from build123d import *

# Parameters (mm, degrees)
F0_W           = 31.095594
F0_H           = 13.626158
F3_D           = 6.35
F3_CSINK_D     = 12.7
F3_CSINK_ANGLE = 90


with BuildPart() as f1:
    # F0 (on Front) → F1 (revolve)
    with BuildSketch(Plane.XZ):
        with Locations((-50.311968, 6.813079)):
            Rectangle(F0_W, F0_H)
    revolve(axis=Axis((0, 0, -5.066134), (0, 0, -1)))

    # F3 (through all)
    with Locations(Plane(origin=(0, 0, 0), x_dir=(1, 0, 0), z_dir=(0, 0, -1))):
        with Locations((55.552796, 0), (0, 55.552796), (-55.552796, 0), (0, -55.552796)):
            CounterSinkHole(F3_D / 2, F3_CSINK_D / 2, counter_sink_angle=F3_CSINK_ANGLE)


solid = f1.part
Input: part model. Units: mm. Frame: model coordinates. Round coordinates to 2 decimals unless told otherwise and drop trailing zeros. Order: outer loops, then holes, each group sorted by start corner. A loop starts at its lowest first (then second) coordinate and runs counter-clockwise, first axis right, second up.
1. Mould query, pull axis Y, two halves, no side actions, for faces 1 (the face through (-28, -28, 0)), 2 (the face through (52.524, -0.954, 8.474)), 3 (the face through (14.277, -64.294, 6.908)). Classes: released by +Y, released by -Y, zero draft, split by the parting line, or undercut.
The answers:
face 1: zero draft
face 2: undercut
face 3: split by the parting line
2. Cut plane D-D, the plane z = 10. Output: boundary loops of the cut face in (x, y) (3 decimals), then the cut area to 3 significant figures.
The answers:
outline: circle Ø131.72 at (0, 0); hole circle Ø6.35 at (-55.553, 0); hole circle Ø69.528 at (0, 0); hole circle Ø6.35 at (0, -55.553); hole circle Ø6.35 at (0, 55.553); hole circle Ø6.35 at (55.553, 0)
area: 9,700 mm2
3. Pin query (flat end, axial travel): P1, Ø6, axis at y = -26.5, z = 6, coming from the +X side; P2, Ø6, axis at y = -43, z = 7, coming from the +X side; P3, Ø5, axis at x = 11.5, z = 10, coming from the +Y side. Return the tip coordinate at first contact, or that it passes through.
The answers:
P1: stops at x = 61.52
P2: stops at x = 52.32
P3: stops at y = 65.24
4. Cut plane A-A, the plane y = 0. Output: boundary loops of the cut face in (x, z) (3 decimals), then the cut area to 3 significant figures.
The answers:
outline: (-65.86, 0) - (-61.903, 0) - (-58.728, 3.175) - (-58.728, 13.626) - (-65.86, 13.626) - close; (-52.378, 3.175) - (-49.203, 0) - (-34.764, 0) - (-34.764, 13.626) - (-52.378, 13.626) - close; (34.764, 0) - (49.203, 0) - (52.378, 3.175) - (52.378, 13.626) - (34.764, 13.626) - close; (58.728, 3.175) - (61.903, 0) - (65.86, 0) - (65.86, 13.626) - (58.728, 13.626) - close
area: 654 mm2
5. Material intervals for line 1 (Y direction, x = 0, z = 11.5); line 2 (Y direction, x = 2.5, z = 11); line 3 (X direction, y = -2, z = 8), sorted ascending.
The answers:
line 1: y = -65.86 to -58.73, -52.38 to -34.76, 34.76 to 52.38, 58.73 to 65.86
line 2: y = -65.81 to -57.51, -53.6 to -34.67, 34.67 to 53.6, 57.51 to 65.81
line 3: x = -65.83 to -58.02, -53.09 to -34.71, 34.71 to 53.09, 58.02 to 65.83
6. Cut plane C-C, the plane x = 23. Output: boundary loops of the cut face in (y, z).
The answers:
outline: (-61.71, 0) - (-26.07, 0) - (-26.07, 13.63) - (-61.71, 13.63) - close; (26.07, 0) - (61.71, 0) - (61.71, 13.63) - (26.07, 13.63) - close
